Check sheet for the drawn part. Datum: minimum x, y, z corner. Units: mm. A direction names the side the tool comes from. Round coordinates to 2 decimals unless told otherwise and drop trailing zeros. Loops run counter-clockwise (first coordinate to the right, second up) from the corner with the lowest first, then second, coordinate; pieces in that order, holes last.
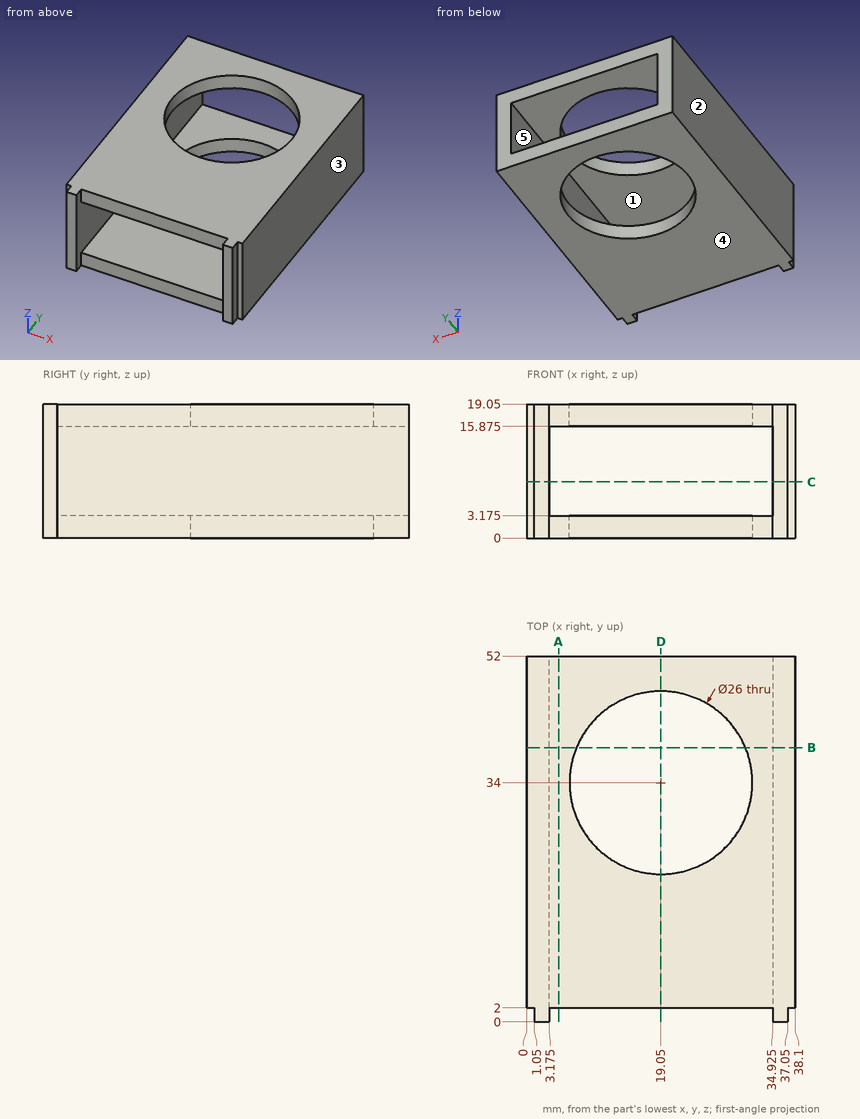
1) Access from +Z, -Z, +X, -X, +Y, -Y to the whole of each face (thin tool, end or side, straight path). Record for the marked faces 1 and 2.
Report:
face 1: +Y, -Y
face 2: +Z, -Z, -X, +Y, -Y
2) Gauge pin test, flat ends, axial feed: pin 1 (0.6 mm diameter, centred on y = 0.5, z = 7.5, fed in from -X); pin 2 (6 mm diameter, centred on x = 14.5, z = 6, fed in from -Y). Record the tip position at first contact, or that the pin passes through.
Report:
pin 1: stops at x = 1.05
pin 2: stops at y = 2
3) Sectioned sample at C-C, the plane z = 8. Record the cut outline in (x, y) (3 decimals), then the cut area to 3 significant figures.
Report:
outline: (0, 2) - (1.05, 2) - (1.05, 0) - (3.175, 0) - (3.175, 52) - (0, 52) - close; (34.925, 0) - (37.05, 0) - (37.05, 2) - (38.1, 2) - (38.1, 52) - (34.925, 52) - close
area: 326 mm2
4) Sectioned sample at B-B, the plane y = 39. Record the cut outline in (x, z) (3 decimals).
Report:
outline: (0, 0) - (7.05, 0) - (7.05, 3.175) - (3.175, 3.175) - (3.175, 15.875) - (7.05, 15.875) - (7.05, 19.05) - (0, 19.05) - close; (31.05, 0) - (38.1, 0) - (38.1, 19.05) - (31.05, 19.05) - (31.05, 15.875) - (34.925, 15.875) - (34.925, 3.175) - (31.05, 3.175) - close
5) Sectioned sample at A-A, the plane x = 4.5. Record the cut outline in (y, z) (3 decimals), then the cut area to 4 significant figures.
Report:
outline: (2, 0) - (52, 0) - (52, 3.175) - (2, 3.175) - close; (2, 15.875) - (52, 15.875) - (52, 19.05) - (2, 19.05) - close
area: 317.5 mm2
6) Sectioned sample at D-D, the plane x = 19.05. Record the cut outline in (y, z) (3 decimals).
Report:
outline: (2, 0) - (21, 0) - (21, 3.175) - (2, 3.175) - close; (2, 15.875) - (21, 15.875) - (21, 19.05) - (2, 19.05) - close; (47, 0) - (52, 0) - (52, 3.175) - (47, 3.175) - close; (47, 15.875) - (52, 15.875) - (52, 19.05) - (47, 19.05) - close
7) Scan lines: line 1 along Z through (x, y) = (28, 45) (3 decimals); line 2 along Y through (x, z) = (19.05, 16.8); line 3 along X through (y, z) = (26, 13) (3 decimals). Record each from-to range of solid material in increasing order.
Report:
line 1: z = 0 to 3.175, 15.875 to 19.05
line 2: y = 2 to 21, 47 to 52
line 3: x = 0 to 3.175, 34.925 to 38.1
8) Mould release check, pull along Z, two halves, no side actions. Record for the marked faces 3, 4 and 5: +Z half, -Z half, draft (parallel to the pull), parting line (faces both ways), or undercut.
Report:
face 3: draft
face 4: -Z half
face 5: undercut
